Design review of the part built by this model. Coordinates are the model's own, in mm. A direction names the side the tool comes from. Give positions to 0.01 mm unless a question says otherwise; leave off trailing zeros. Write each loop counter-clockwise with the first axis right and the second up, starting at its lowest first coordinate (ties: lowest second). Pieces come first, ordered by that corner, then holes. Notation, with made-up numbers: M 57,52.5 L 104,52.5 A12 ccw 104,66.5 Z; hole C 87.25,18.25 d10. An arc over 180 degrees is marked long. Use a Markdown table: item, result. Add a question column.
```python
from build123d import *

# Parameters (mm, degrees)
F0_R     = 1.25
F1_DEPTH = 1.2
F2_R     = 2.5
F3_DEPTH = 2


with BuildPart() as f1:
    # F0 (on Top) → F1 (new body)
    with BuildSketch(Plane.XY):
        with BuildLine():
            Line((14.086174, 1.998143), (2.44949, 2.5))
            ThreePointArc((2.44949, 2.5), (-3.5, 0), (2.44949, -2.5))
            Line((2.44949, -2.5), (14.086174, -1.998143))
            ThreePointArc((14.086174, -1.998143), (16, 0), (14.086174, 1.998143))
        make_face()
        Circle(F0_R, mode=Mode.SUBTRACT)
    extrude(amount=F1_DEPTH)

    # F2 (on face) → F3 (join)
    with BuildSketch(Plane.XY.offset(1.2)):
        with BuildLine():
            ThreePointArc((2.44949, -2.5), (3.226702, -1.355874), (3.5, 0))
            ThreePointArc((3.5, 0), (3.226702, 1.355874), (2.44949, 2.5))
            ThreePointArc((2.44949, 2.5), (-3.5, 0), (2.44949, -2.5))
        make_face()
        Circle(F2_R, mode=Mode.SUBTRACT)
    extrude(amount=F3_DEPTH)


solid = f1.part
```
(1) Add section C-C on z = 0.7. Give the boundary of the cut face in (x, y), then the cut area to 3 significant figures.
(2) Machinability: for faces 1 (the flat face through (-1, -1, 1.2)), 2 (the flat face through (8.349, 2.246, 0.592)), which of the approach directions +Z, -Z, +X, -X, +Y, -Y give a long, thin tool a straight path to every point of the face, cutting with its end or side? Answer none if there is none.
(3) The part is to be moulded in two halves that separate along Y. For faces 3 (the cylindrical face through (-0.54, -2.44, 2.19)), 4 (the cylindrical face through (16, 0, 1)), 5 (the flat face through (2, -2, 3.2)), say which applies: released by +Y, released by -Y, zero draft, split by the parting line, or undercut.
(4) For pin 1 (1.5 mm diameter, centred on x = 8.5, y = -0.5, fed in from +Z); pin 2 (1.5 mm diameter, centred on x = 13.5, z = 0.5, fed in from -Y), all flat-tipped, find the tip position at first contact; note any pin that passes through.
(5) Wall thickness on L1, parallel to Y at x = 0, z = 2.1; L2, parallel to Y at x = 1.5, z = 2.1; L3, parallel to Z at x = 5.5, y = -0.75: over which ranges is each line inside the solid? List them lowest first.
(6) Add section B-B on y = -1. Give the boundary of the cut face in (x, z), then the cut area to 3 significant figures.
(7) Add section A-A on x = 0. Give the boundary of the cut face in (y, z), then the cut area to 3 significant figures.
(8) Add section D-D on y = -2.25. Give the boundary of the cut face in (x, z), then the cut area to 3 significant figures.
From the geometry:
| question | item | result |
|---|---|---|
| 1 | outline | M 2.45,-2.5 L 14.09,-2 A2 ccw 14.09,2 L 2.45,2.5 A3.5 ccw long Z; hole C 0,0 d2.5 |
| 1 | area | 88.2 mm^2 |
| 2 | face 1 | +Z |
| 2 | face 2 | +Z, -Z, +X, +Y |
| 3 | face 3 | undercut |
| 3 | face 4 | split by the parting line |
| 3 | face 5 | zero draft |
| 4 | pin 1 | stops at z = 1.2 |
| 4 | pin 2 | stops at y = -2.06 |
| 5 | L1 | y = -3.5 to -2.5, 2.5 to 3.5 |
| 5 | L2 | y = -3.16 to -2, 2 to 3.16 |
| 5 | L3 | z = 0 to 1.2 |
| 6 | outline | M -3.35,0 L -0.75,0 L -0.75,1.2 L -2.29,1.2 L -2.29,3.2 L -3.35,3.2 Z; M 0.75,0 L 15.73,0 L 15.73,1.2 L 3.35,1.2 L 3.35,3.2 L 2.29,3.2 L 2.29,1.2 L 0.75,1.2 Z |
| 6 | area | 25.4 mm^2 |
| 7 | outline | M -3.5,0 L -1.25,0 L -1.25,1.2 L -2.5,1.2 L -2.5,3.2 L -3.5,3.2 Z; M 1.25,0 L 3.5,0 L 3.5,3.2 L 2.5,3.2 L 2.5,1.2 L 1.25,1.2 Z |
| 7 | area | 9.40 mm^2 |
| 8 | outline | M -2.68,0 L 8.25,0 L 8.25,1.2 L 2.68,1.2 L 2.68,3.2 L 1.09,3.2 L 1.09,1.2 L -1.09,1.2 L -1.09,3.2 L -2.68,3.2 Z |
| 8 | area | 19.5 mm^2 |
